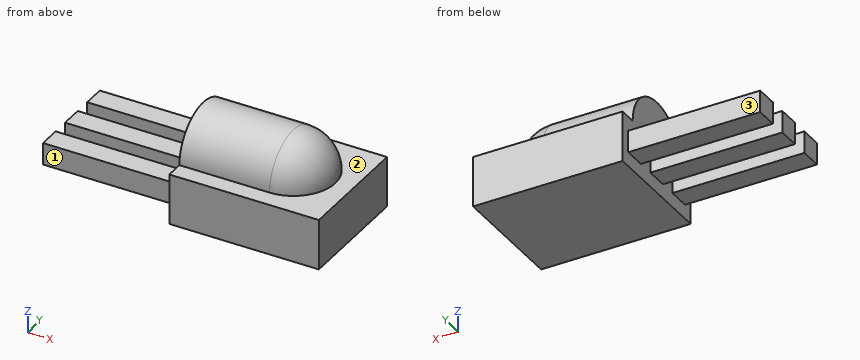
from build123d import *

# Parameters (mm, degrees)
ESQUISSE1_W        = 6.8
ESQUISSE1_H        = 5.4
BOSS_EXTRU_1_DEPTH = 2.3
ESQUISSE2_R        = 1.9
BOSS_EXTRU_2_DEPTH = 6
CONG_1_R           = 1.9
ESQUISSE3_W        = 1
ESQUISSE3_H        = 1
BOSS_EXTRU_3_DEPTH = 6


with BuildPart() as part:
    # Esquisse1 → Boss.-Extru.1 (new body)
    with BuildSketch(Plane.XY):
        with Locations((3.4, 2.7)):
            Rectangle(ESQUISSE1_W, ESQUISSE1_H)
    extrude(amount=BOSS_EXTRU_1_DEPTH)

    # Esquisse2 → Boss.-Extru.2 (add)
    with BuildSketch(Plane.ZY):
        with Locations((2.3, 2.7)):
            Circle(ESQUISSE2_R)
    extrude(amount=-BOSS_EXTRU_2_DEPTH)

    # Congé1
    cong_1_edges = [part.edges().sort_by_distance(p)[0] for p in [
        (6, 2.7, 4.2),
    ]]
    fillet(cong_1_edges, radius=CONG_1_R - 0.0001)  # a hair under: the kernel refuses the full size

    # Esquisse3 → Boss.-Extru.3 (add)
    with BuildSketch(Plane.ZY):
        with Locations((1.15, 4.45)):
            Rectangle(ESQUISSE3_W, ESQUISSE3_H)
        with Locations((1.15, 2.7)):
            Rectangle(ESQUISSE3_W, ESQUISSE3_H)
        with Locations((1.15, 0.95)):
            Rectangle(ESQUISSE3_W, ESQUISSE3_H)
    extrude(amount=BOSS_EXTRU_3_DEPTH)


solid = part.part
Verification items for the finished model (mm, model axes). Face numbers are marked on the shaded views. A direction names the side the tool comes from. Give positions to 0.01 mm unless a question says otherwise; leave off trailing zeros. Order: outer loops, then holes, each group sorted by start corner. A loop starts at its lowest first (then second) coordinate and runs counter-clockwise, first axis right, second up. Notation, with made-up numbers: M 83,-4 L 123,-4 A10 ccw 123,0 Z; hole C 8.25,22.25 d3. An arc over 180 degrees is marked long. Use one line per item in the form item = value. Start each with the question number.
Q1. Section check A-A (x = -0.75). Enter the section's corners in (y, z).
Q2. Access from +Z, -Z, +X, -X, +Y, -Y to the whole of each face (thin tool, end or side, straight path). Record for the marked faces 1, 2 and 3.
Q3. Scan lines: line 1 along Y through (x, z) = (-1.25, 1.15); line 2 along X through (y, z) = (1.5, 1.15); line 3 along Z through (x, y) = (-3, 4.85). Record each from-to range of solid material in increasing order. Write a range as [from, to].
Q4. Go/stop test with flat-tipped pins: pin 1 Ø1.5 at (x, y) = (-4, 1.5) entering from -Z; pin 2 Ø0.8 at (x, z) = (-3, 1) entering from -Y; pin 3 Ø1.1 at (x, y) = (-2.5, 1) entering from +Z. Record where each tip stops, or that it passes through.
Q5. Section check B-B (z = 1.25). Enter the section's corners in (x, y), then the cut area to 3 significant figures.
Evaluation:
q1.outline = M 0.45,0.65 L 1.45,0.65 L 1.45,1.65 L 0.45,1.65 Z; M 2.2,0.65 L 3.2,0.65 L 3.2,1.65 L 2.2,1.65 Z; M 3.95,0.65 L 4.95,0.65 L 4.95,1.65 L 3.95,1.65 Z
q2.face_1 = +Z, -Z, -X, -Y
q2.face_2 = +Z, +X
q2.face_3 = +Z, -Z, -X, +Y
q3.line_1 = [0.45, 1.45], [2.2, 3.2], [3.95, 4.95]
q3.line_2 = [0, 6.8]
q3.line_3 = [0.65, 1.65]
q4.pin_1 = 0.65
q4.pin_2 = 0.45
q4.pin_3 = 1.65
q5.outline = M -6,0.45 L 0,0.45 L 0,0 L 6.8,0 L 6.8,5.4 L 0,5.4 L 0,4.95 L -6,4.95 L -6,3.95 L 0,3.95 L 0,3.2 L -6,3.2 L -6,2.2 L 0,2.2 L 0,1.45 L -6,1.45 Z
q5.area = 54.7 mm2
